Part model, mm, in its own coordinate system. A direction names the side the tool comes from. Round coordinates to 2 decimals unless told otherwise and drop trailing zeros. Write each loop counter-clockwise with the first axis right and the second up, starting at its lowest first coordinate (ties: lowest second). Pieces come first, ordered by that corner, then holes.
1) Which spindle directions (+Z, -Z, +X, -X, +Y, -Y) get a long thin tool onto all of the face, cutting with end or side? Do faces 1 (the flat face through (-10, -13, 139)), 2 (the flat face through (77, 12, 31)), 3 (the flat face through (9, -10, 139)). Say none if no direction does.
2) Drill centre lines: L1, parallel to X at y = 18, z = 60.5; L2, parallel to Z at x = 31, y = 14. Where is each one in solid material? Low to high.
3) Pull direction X, two halves, no side cores. Call faces 4 (the flat face through (66, -16, 139)), 5 (the flat face through (-1, -20, 73)), 6 (the flat face through (-76, 1, 73)): +X half, -X half, draft (parallel to the pull), parting line (faces both ways), or undercut.
4) Flat gauge pins, fed straight in: pin 1 (7.5 mm diameter, centred on x = 67, z = 136.5, fed in from +Y); pin 2 (12 mm diameter, centred on y = -9.5, z = 139.5, fed in from +X); pin 3 (8 mm diameter, centred on x = -26, y = 1.5, fed in from +Z); pin 4 (0.6 mm diameter, centred on x = -4, y = -15, fed in from -Z). Where does each tip first touch, or does it go through?
5) Saw through at A-A on x = -5.5. Write the cut outline in (y, z), and give its area (3 significant figures).
```python
from build123d import *

# Parameters (mm, degrees)
SKETCH1_W           = 152
SKETCH1_H           = 40
BOSS_EXTRUDE1_DEPTH = 132
SKETCH2_W           = 152
SKETCH2_H           = 132
BOSS_EXTRUDE2_DEPTH = 3
SKETCH4_W           = 20
SKETCH4_H           = 20
BOSS_EXTRUDE3_DEPTH = 16
SKETCH7_W           = 18
SKETCH7_H           = 15
CUT_EXTRUDE1_DEPTH  = 16
CUT_EXTRUDE2_DEPTH  = 214.39400179
FILLET1_R           = 1
SKETCH9_W           = 22
SKETCH9_H           = 10
SKETCH9_W_2         = 52
SKETCH9_H_2         = 8
BOSS_EXTRUDE4_DEPTH = 1


with BuildPart() as part:
    # Sketch1 → Boss-Extrude1 (new body)
    with BuildSketch(Plane.XY):
        Rectangle(SKETCH1_W, SKETCH1_H)
    extrude(amount=BOSS_EXTRUDE1_DEPTH)

    # Sketch2 → Boss-Extrude2 (add)
    with BuildSketch(Plane(origin=(0, 20, 0), x_dir=(1, 0, 0), z_dir=(0, 1, 0))):
        with Locations((0, -66)):
            Rectangle(SKETCH2_W, SKETCH2_H)
    extrude(amount=BOSS_EXTRUDE2_DEPTH)

    # Sketch4 → Boss-Extrude3 (add)
    with BuildSketch(Plane.XY.offset(132)):
        with Locations((-66, -10)):
            Rectangle(SKETCH4_W, SKETCH4_H)
        with Locations((66, -10)):
            Rectangle(SKETCH4_W, SKETCH4_H)
        with Locations((0, -10)):
            Rectangle(SKETCH4_W, SKETCH4_H)
    extrude(amount=BOSS_EXTRUDE3_DEPTH)

    # Sketch7 → Cut-Extrude1 (cut)
    with BuildSketch(Plane(origin=(0, 0, 0), x_dir=(1, 0, 0), z_dir=(0, 1, 0))):
        with Locations((66, -139.5)):
            Rectangle(SKETCH7_W, SKETCH7_H)
        with Locations((0, -139.5)):
            Rectangle(SKETCH7_W, SKETCH7_H)
        with Locations((-66, -139.5)):
            Rectangle(SKETCH7_W, SKETCH7_H)
    extrude(amount=-CUT_EXTRUDE1_DEPTH, mode=Mode.SUBTRACT)

    # Sketch8 → Cut-Extrude2 (cut, through all)
    with BuildSketch(Plane(origin=(76, 0, 0), x_dir=(0, 0, -1), z_dir=(1, 0, 0))):
        Polygon((-132, 0), (-148, -15), (-148, 0), align=None)
    extrude(amount=-CUT_EXTRUDE2_DEPTH, mode=Mode.SUBTRACT)

    # Fillet1
    fillet1_edges = [part.edges().sort_by_distance(p)[0] for p in [
        (-56, -10, 132),
        (56, -10, 132),
        (-10, -10, 132),
        (10, -10, 132),
        (57, -8, 132),
        (75, -8, 132),
        (-9, -8, 132),
        (9, -8, 132),
        (-75, -8, 132),
        (-57, -8, 132),
    ]]
    fillet(fillet1_edges, radius=FILLET1_R)

    # Sketch9 → Boss-Extrude4 (add)
    with BuildSketch(Plane(origin=(76, 0, 0), x_dir=(0, 0, -1), z_dir=(1, 0, 0))):
        with Locations((-99, 13)):
            Rectangle(SKETCH9_W, SKETCH9_H)
        with Locations((-31, 12)):
            Rectangle(SKETCH9_W_2, SKETCH9_H_2)
    extrude(amount=BOSS_EXTRUDE4_DEPTH)


solid = part.part
```
Completed:
1. face 1: +Z, +Y, -Y
1. face 2: +Z, -Z, +X, +Y, -Y
1. face 3: +Y
2. L1: x = -76 to 76
2. L2: z = 0 to 132
3. face 4: undercut
3. face 5: draft
3. face 6: -X half
4. pin 1: stops at y = -16
4. pin 2: stops at x = 76
4. pin 3: stops at z = 132
4. pin 4: stops at z = 0
5. outline: (-20, 0) - (23, 0) - (23, 132) - (-16, 132) - (-16, 147) - (-14.06, 147) - (-15, 148) - (-20, 148) - close
5. area: 5,740 mm2
